from build123d import *

# Parameters (mm, degrees)
SKETCH1_R           = 40.5
SKETCH1_R_2         = 1.5
BOSS_EXTRUDE1_DEPTH = 3


with BuildPart() as part:
    # Sketch1 → Boss-Extrude1 (new body)
    with BuildSketch(Plane(origin=(0, 0, 0), x_dir=(1, 0, 0), z_dir=(0, 1, 0))):
        with Locations(Location((0, 0, 0), (0, 0, 270))):
            Circle(SKETCH1_R)
        with Locations(Location((-13.447058678, 23.290988922, 0), (0, 0, 270))):
            Circle(SKETCH1_R_2, mode=Mode.SUBTRACT)
        with Locations(Location((26.894117425, -4e-08, 0), (0, 0, 270))):
            Circle(SKETCH1_R_2, mode=Mode.SUBTRACT)
        with Locations(Location((-13.447058747, -23.290988882, 0), (0, 0, 270))):
            Circle(SKETCH1_R_2, mode=Mode.SUBTRACT)
        with BuildLine():
            Line((6.085843699, 27.540990494), (2.560351484, 21.434658856))
            ThreePointArc((2.560351484, 21.434658856), (0.888284255, 19.699718697), (-1.401072298, 18.948271594))
            ThreePointArc((-1.401072298, 18.948271594), (-9.5, 16.454482672), (-15.709148409, 10.6875))
            ThreePointArc((-15.709148409, 10.6875), (-17.504598966, 9.080582618), (-19.843134833, 8.5))
            Line((-19.843134833, 8.5), (-26.894119263, 8.5))
            ThreePointArc((-26.894119263, 8.5), (-35.394119263, 0), (-26.894119263, -8.5))
            Line((-26.894119263, -8.5), (-19.843134833, -8.5))
            ThreePointArc((-19.843134833, -8.5), (-17.504598966, -9.080582618), (-15.709148409, -10.6875))
            ThreePointArc((-15.709148409, -10.6875), (-9.5, -16.454482672), (-1.401072298, -18.948271594))
            ThreePointArc((-1.401072298, -18.948271594), (0.888284255, -19.699718697), (2.560351484, -21.434658856))
            Line((2.560351484, -21.434658856), (6.085843699, -27.540990494))
            ThreePointArc((6.085843699, -27.540990494), (17.697059631, -30.652206426), (20.808275564, -19.040990494))
            Line((20.808275564, -19.040990494), (17.282783349, -12.934658856))
            ThreePointArc((17.282783349, -12.934658856), (16.616314711, -10.619136079), (17.110220708, -8.260771594))
            ThreePointArc((17.110220708, -8.260771594), (19, 0), (17.110220708, 8.260771594))
            ThreePointArc((17.110220708, 8.260771594), (16.616314711, 10.619136079), (17.282783349, 12.934658856))
            Line((17.282783349, 12.934658856), (20.808275564, 19.040990494))
            ThreePointArc((20.808275564, 19.040990494), (17.697059631, 30.652206426), (6.085843699, 27.540990494))
        make_face(mode=Mode.SUBTRACT)
    extrude(amount=-BOSS_EXTRUDE1_DEPTH)


solid = part.part
Could you check a few things on this model? Use its own coordinates, in mm. A direction names the side the tool comes from. Give positions to 0.01 mm unless a question says otherwise; leave off trailing zeros. Order: outer loops, then holes, each group sorted by start corner. A loop starts at its lowest first (then second) coordinate and runs counter-clockwise, first axis right, second up.
Item 1: I'm going to push flat-ended pins straight in: pin 1 (2.5 mm diameter, centred on x = -13.45, z = -23.29, fed in from -Y); pin 2 (1.5 mm diameter, centred on x = -12, y = -1.5, fed in from -Z). Where does each tip first touch, or does it pass through?
Item 2: If we section it at C-C, the plane z = 20: Write out the boundary of the cut face in (x, y), plus the area to 3 significant figures.
Item 3: I need wall thicknesses on line 1 (X direction, y = -1.4, z = 0); line 2 (X direction, y = -2.6, z = -23); line 3 (Z direction, x = 17, y = -0.45). Which ranges of each line are inside material? Lowest first, please.
Item 4: If we mould it in two halves opening along Z, with no side actions, what happens to faces 3 (the face through (-8.4, 0, 17.4)), 4 (the face through (34.15, -1.48, 21.77)), 5 (the face through (-17.535, -1.479, 9.065))? For each: pulls with the +Z half, pulls with the -Z half, needs draft (parallel to the pull), parting line crosses it, or undercut.
Item 5: If we section it at D-D, the plane y = -1.55: Write out the boundary of the cut face in (x, z), plus the area to 3 significant figures.
Item 6: If we section it at A-A, the plane z = 0: Write out the boundary of the cut face in (x, y), plus the area to 3 significant figures.
Item 7: If we section it at B-B, the plane x = -33.5: Write out the boundary of the cut face in (y, z).
Item 8: For faces 1 (the face through (-8.4, -3, 17.4)), 2 (the face through (16.618, -1.479, 10.653)), which set-ups out of +Z, -Z, +X, -X, +Y, -Y let a thin tool reach every point of the face, with its end or its side?
Values:
1. pin 1: passes through
1. pin 2: stops at z = -38.91
2. outline: (-35.22, -3) - (1.32, -3) - (1.32, 0) - (-35.22, 0) - close; (21.28, -3) - (35.22, -3) - (35.22, 0) - (21.28, 0) - close
2. area: 151 mm2
3. line 1: x = -40.5 to -35.39, 19 to 25.39, 28.39 to 40.5
3. line 2: x = -33.34 to -14.92, -11.98 to 3.46, 21.94 to 33.34
3. line 3: z = -36.76 to -31.01, -12.36 to -8.51, 8.51 to 12.36, 31.01 to 36.76
4. face 3: needs draft
4. face 4: parting line crosses it
4. face 5: undercut
5. outline: circle Ø81 at (0, 0); hole (-26.89, -8.5) - (-19.84, -8.5) arc R5 cw to (-15.71, -10.69) arc R19 ccw to (-1.4, -18.95) arc R5 cw to (2.56, -21.43) - (6.09, -27.54) arc R8.5 ccw to (20.81, -19.04) - (17.28, -12.93) arc R5 cw to (17.11, -8.26) arc R19 ccw to (17.11, 8.26) arc R5 cw to (17.28, 12.93) - (20.81, 19.04) arc R8.5 ccw to (6.09, 27.54) - (2.56, 21.43) arc R5 cw to (-1.4, 18.95) arc R19 ccw to (-15.71, 10.69) arc R5 cw to (-19.84, 8.5) - (-26.89, 8.5) arc R8.5 ccw to start; hole circle Ø3 at (-13.45, -23.29); hole circle Ø3 at (-13.45, 23.29); hole circle Ø3 at (26.89, 0)
5. area: 3,210 mm2
6. outline: (-40.5, -3) - (-35.39, -3) - (-35.39, 0) - (-40.5, 0) - close; (19, -3) - (25.39, -3) - (25.39, 0) - (19, 0) - close; (28.39, -3) - (40.5, -3) - (40.5, 0) - (28.39, 0) - close
6. area: 70.8 mm2
7. outline: (-3, -22.76) - (0, -22.76) - (0, -5.35) - (-3, -5.35) - close; (-3, 5.35) - (0, 5.35) - (0, 22.76) - (-3, 22.76) - close
8. face 1: +Z, -Z, +X, -X, -Y
8. face 2: +Y, -Y
